```python
from build123d import *

# Parameters (mm, degrees)
EXTRUSION1_DEPTH = 47
ESQUISSE2_R      = 2
ESQUISSE2_W      = 3
ESQUISSE2_H      = 48
EXTRUSION2_DEPTH = 59
EXTRUSION3_REACH = 60
ESQUISSE3_R      = 2
EXTRUSION4_DEPTH = 5


with BuildPart() as part:
    # Esquisse1 → Extrusion1 (new body)
    with BuildSketch(Plane.XY):
        Polygon((0, -20), (0, 37.5), (46, 37.5), (46, -20), (54, -20), (54, 41.5), (-4, 41.5), (-4, -20), align=None)
    extrude(amount=EXTRUSION1_DEPTH)

    # Esquisse2 → Extrusion2 (cut, through all)
    with BuildSketch(Plane(origin=(54, 0, 0), x_dir=(0, 0, -1), z_dir=(1, 0, 0))):
        with Locations((-24, 0)):
            Circle(ESQUISSE2_R)
        with Locations((-1.5, 13.5)):
            Rectangle(ESQUISSE2_W, ESQUISSE2_H)
    extrude(amount=-EXTRUSION2_DEPTH, mode=Mode.SUBTRACT)

    # Esquisse3 → Extrusion3 (cut, up to next)
    with BuildSketch(Plane(origin=(54, 0, 0), x_dir=(0, 0, -1), z_dir=(1, 0, 0)), mode=Mode.PRIVATE) as extrusion3_sk1:
        with Locations((-24, 14)):
            Circle(ESQUISSE3_R)
    extrusion3_tool1 = extrude(extrusion3_sk1.sketch, amount=-EXTRUSION3_REACH, mode=Mode.PRIVATE) & part.part
    add(extrusion3_tool1.solids().sort_by_distance((54, 14, 24))[0], mode=Mode.SUBTRACT)
    # Esquisse3 → Extrusion3 (cut, up to next)
    with BuildSketch(Plane(origin=(54, 0, 0), x_dir=(0, 0, -1), z_dir=(1, 0, 0)), mode=Mode.PRIVATE) as extrusion3_sk2:
        with Locations((-14.100505063, 9.899494937)):
            Circle(ESQUISSE3_R)
    extrusion3_tool2 = extrude(extrusion3_sk2.sketch, amount=-EXTRUSION3_REACH, mode=Mode.PRIVATE) & part.part
    add(extrusion3_tool2.solids().sort_by_distance((54, 9.899495, 14.100505))[0], mode=Mode.SUBTRACT)
    # Esquisse3 → Extrusion3 (cut, up to next)
    with BuildSketch(Plane(origin=(54, 0, 0), x_dir=(0, 0, -1), z_dir=(1, 0, 0)), mode=Mode.PRIVATE) as extrusion3_sk3:
        with Locations((-10, 0)):
            Circle(ESQUISSE3_R)
    extrusion3_tool3 = extrude(extrusion3_sk3.sketch, amount=-EXTRUSION3_REACH, mode=Mode.PRIVATE) & part.part
    add(extrusion3_tool3.solids().sort_by_distance((54, 0, 10))[0], mode=Mode.SUBTRACT)
    # Esquisse3 → Extrusion3 (cut, up to next)
    with BuildSketch(Plane(origin=(54, 0, 0), x_dir=(0, 0, -1), z_dir=(1, 0, 0)), mode=Mode.PRIVATE) as extrusion3_sk4:
        with Locations((-14.100505063, -9.899494937)):
            Circle(ESQUISSE3_R)
    extrusion3_tool4 = extrude(extrusion3_sk4.sketch, amount=-EXTRUSION3_REACH, mode=Mode.PRIVATE) & part.part
    add(extrusion3_tool4.solids().sort_by_distance((54, -9.899495, 14.100505))[0], mode=Mode.SUBTRACT)
    # Esquisse3 → Extrusion3 (cut, up to next)
    with BuildSketch(Plane(origin=(54, 0, 0), x_dir=(0, 0, -1), z_dir=(1, 0, 0)), mode=Mode.PRIVATE) as extrusion3_sk5:
        with Locations((-24, -14)):
            Circle(ESQUISSE3_R)
    extrusion3_tool5 = extrude(extrusion3_sk5.sketch, amount=-EXTRUSION3_REACH, mode=Mode.PRIVATE) & part.part
    add(extrusion3_tool5.solids().sort_by_distance((54, -14, 24))[0], mode=Mode.SUBTRACT)
    # Esquisse3 → Extrusion3 (cut, up to next)
    with BuildSketch(Plane(origin=(54, 0, 0), x_dir=(0, 0, -1), z_dir=(1, 0, 0)), mode=Mode.PRIVATE) as extrusion3_sk6:
        with Locations((-33.899494937, -9.899494937)):
            Circle(ESQUISSE3_R)
    extrusion3_tool6 = extrude(extrusion3_sk6.sketch, amount=-EXTRUSION3_REACH, mode=Mode.PRIVATE) & part.part
    add(extrusion3_tool6.solids().sort_by_distance((54, -9.899495, 33.899495))[0], mode=Mode.SUBTRACT)
    # Esquisse3 → Extrusion3 (cut, up to next)
    with BuildSketch(Plane(origin=(54, 0, 0), x_dir=(0, 0, -1), z_dir=(1, 0, 0)), mode=Mode.PRIVATE) as extrusion3_sk7:
        with Locations((-38, 0)):
            Circle(ESQUISSE3_R)
    extrusion3_tool7 = extrude(extrusion3_sk7.sketch, amount=-EXTRUSION3_REACH, mode=Mode.PRIVATE) & part.part
    add(extrusion3_tool7.solids().sort_by_distance((54, 0, 38))[0], mode=Mode.SUBTRACT)
    # Esquisse3 → Extrusion3 (cut, up to next)
    with BuildSketch(Plane(origin=(54, 0, 0), x_dir=(0, 0, -1), z_dir=(1, 0, 0)), mode=Mode.PRIVATE) as extrusion3_sk8:
        with Locations((-33.899494937, 9.899494937)):
            Circle(ESQUISSE3_R)
    extrusion3_tool8 = extrude(extrusion3_sk8.sketch, amount=-EXTRUSION3_REACH, mode=Mode.PRIVATE) & part.part
    add(extrusion3_tool8.solids().sort_by_distance((54, 9.899495, 33.899495))[0], mode=Mode.SUBTRACT)

    # Esquisse4 → Extrusion4 (cut, through all)
    with BuildSketch(Plane.XZ.offset(-37.5)):
        Polygon((5, 47), (5, 29), (23, 29), (23, 38), (46, 38), (46, 47), (23, 47), align=None)
    extrude(amount=-EXTRUSION4_DEPTH, mode=Mode.SUBTRACT)


solid = part.part
```
CAD build for the part. Positions are in the model's coordinates, mm. A direction names the side the tool comes from. Round coordinates to 2 decimals unless told otherwise and drop trailing zeros. Write each loop counter-clockwise with the first axis right and the second up, starting at its lowest first coordinate (ties: lowest second). Pieces come first, ordered by that corner, then holes. Notation, with made-up numbers: (55.5, -27.5) - (100.5, -27.5) arc R11 cw to (100.5, -8.5) - close; hole circle Ø8 at (27.5, 2). An arc over 180 degrees is marked (long way). Write item = value, one per line. Start each with the question number.
Q1. Drop flat-ended pins along their axis: pin 1 (3 mm diameter, centred on y = 0, z = 24, fed in from -X); pin 2 (14 mm diameter, centred on x = 36.5, z = 16.5, fed in from -Y); pin 3 (3.5 mm diameter, centred on y = -9.9, z = 33.9, fed in from +X). Give the stop position or say it passes through.
Q2. Mould opens along X. For faces 1 (the flat face through (25, 37.5, 18)), 2 (the flat face through (-2, -15, 0)) say: pulls with the +X half, pulls with the -X half, needs draft (parallel to the pull), parting line crosses it, or undercut.
Q3. Band-saw the part on A-A (z = 10). Give the cut face in (x, y).
Q4. Band-saw the part on D-D (y = -14). Give the cut face in (x, z), then the cut area to 3 significant figures.
Q5. Band-saw the part on B-B (y = 20). Give the cut face in (x, z), then the cut area to 3 significant figures.
Q6. Which spindle directions (+Z, -Z, +X, -X, +Y, -Y) get a long thin tool onto all of the face, cutting with end or side? Do faces 3 (the flat face through (0, 8, 23)), 4 (the flat face through (-2, 13, 3)), 5 (the flat face through (50, -20, 23)), 6 (the cylindrical face through (50.056, 10.5, 12.193)), 7 (the flat face through (14, 39, 29)). Say none if no direction does.
Q7. Probe L1, parallel to Y at x = 50.25, z = 24; L2, parallel to X at y = 18.5, z = 9; L3, parallel to Y at x = -2.05, z = 24. List the from-to ranges inside material, lowest first. Write a range as from..to.
Q8. Band-saw the part on C-C (z = 24). Give the cut face in (x, y), then the cut area to 3 significant figures.
Answers below:
q1.pin_1 = through
q1.pin_2 = 37.5
q1.pin_3 = 0
q2.face_1 = undercut
q2.face_2 = needs draft
q3.outline = (-4, -20) - (0, -20) - (0, 37.5) - (46, 37.5) - (46, 2) - (54, 2) - (54, 41.5) - (-4, 41.5) - close; (46, -20) - (54, -20) - (54, -2) - (46, -2) - close
q4.outline = (-4, 0) - (0, 0) - (0, 47) - (-4, 47) - close; (46, 0) - (54, 0) - (54, 22) - (46, 22) - close; (46, 26) - (54, 26) - (54, 47) - (46, 47) - close
q4.area = 532 mm2
q5.outline = (-4, 3) - (0, 3) - (0, 47) - (-4, 47) - close; (46, 3) - (54, 3) - (54, 47) - (46, 47) - close
q5.area = 528 mm2
q6.face_3 = +Z, -Z, -Y
q6.face_4 = -Z, +X, -X
q6.face_5 = +Z, -Z, +X, -X, -Y
q6.face_6 = +X
q6.face_7 = +Z, +Y, -Y
q7.L1 = -20..-16, -12..-2, 2..12, 16..41.5
q7.L2 = -4..0, 46..54
q7.L3 = -20..-2, 2..41.5
q8.outline = (-4, -20) - (0, -20) - (0, -2) - (-4, -2) - close; (-4, 2) - (0, 2) - (0, 37.5) - (46, 37.5) - (46, 16) - (54, 16) - (54, 41.5) - (-4, 41.5) - close; (46, -20) - (54, -20) - (54, -16) - (46, -16) - close; (46, -12) - (54, -12) - (54, -2) - (46, -2) - close; (46, 2) - (54, 2) - (54, 12) - (46, 12) - close
q8.area = 810 mm2
